Design review of the part built by this model. Coordinates are the model's own, in mm. A direction names the side the tool comes from. Give positions to 0.01 mm unless a question says otherwise; leave off trailing zeros. Loops run counter-clockwise (first coordinate to the right, second up) from the corner with the lowest first, then second, coordinate; pieces in that order, holes last. Notation, with made-up numbers: M 15,73 L 70,73 A21 ccw 70,87 Z; hole C 13.5,73.5 d11. An arc over 180 degrees is marked long. Answer as CSV lines item,"result".
```python
from build123d import *
from build123d.topology import SkipClean

# Parameters (mm, degrees)
SKETCH2_R               = 15
SKETCH2_R_2             = 11.15
BOSS_EXTRUDE1_DEPTH     = 7
SKETCH3_R               = 15
SKETCH3_R_2             = 9
BOSS_EXTRUDE2_DEPTH     = 3
BOSS_EXTRUDE3_START     = 5
SKETCH4_R               = 15
SKETCH4_R_2             = 11.15
BOSS_EXTRUDE3_DEPTH     = 5
BOSS_EXTRUDE4_DEPTH     = 8
BOSS_EXTRUDE5_START     = 20
SKETCH7_W               = 10
SKETCH7_H               = 30
BOSS_EXTRUDE5_DEPTH     = 20
BOSS_EXTRUDE6_DEPTH     = 7
SKETCH10_W              = 2
SKETCH10_H              = 90
CUT_EXTRUDE1_DEPTH      = 20
SKETCH12_R              = 2.75
CUT_EXTRUDE2_DEPTH      = 20
BOSS_EXTRUDE7_DEPTH     = 10
BOSS_EXTRUDE8_DEPTH     = 10
SKETCH15_W              = 10
SKETCH15_H              = 10
BOSS_EXTRUDE9_DEPTH     = 20
SKETCH16_W              = 10
SKETCH16_H              = 10
BOSS_EXTRUDE10_DEPTH    = 10
SKETCH17_W              = 10
SKETCH17_H              = 10
BOSS_EXTRUDE11_DEPTH    = 90
FILLET1_R               = 7.5
BOSS_EXTRUDE12_START    = 10
SKETCH18_R              = 11.15
BOSS_EXTRUDE12_DEPTH    = 10
BOSS_EXTRUDE13_START    = -3
SKETCH19_R              = 9
BOSS_EXTRUDE13_DEPTH    = 3
CUT_EXTRUDE3_DEPTH      = 88.943163464
CUT_EXTRUDE3_DEPTH_BACK = 88.943163464
SKETCH21_W              = 10
SKETCH21_H              = 10
BOSS_EXTRUDE14_DEPTH    = 20
SKETCH22_W              = 10
SKETCH22_H              = 20
BOSS_EXTRUDE15_DEPTH    = 20
FILLET2_R               = 7.5
SKETCH23_R              = 2.75
CUT_EXTRUDE4_DEPTH      = 20


with BuildPart() as part:
    # Sketch2 → Boss-Extrude1 (new body)
    with BuildSketch(Plane.XY):
        Circle(SKETCH2_R)
        Circle(SKETCH2_R_2, mode=Mode.SUBTRACT)
    extrude(amount=-BOSS_EXTRUDE1_DEPTH)

    # Sketch3 → Boss-Extrude2 (add)
    with BuildSketch(Plane(origin=(0, 0, -7), x_dir=(-1, 0, 0), z_dir=(0, 0, -1))):
        with Locations(Location((0, 0, 0), (0, 0, 180))):
            Circle(SKETCH3_R)
        Circle(SKETCH3_R_2, mode=Mode.SUBTRACT)
    extrude(amount=BOSS_EXTRUDE2_DEPTH)

    # Sketch4 → Boss-Extrude3 (add)
    with BuildSketch(Plane.XY.offset(BOSS_EXTRUDE3_START)):
        Circle(SKETCH4_R)
        Circle(SKETCH4_R_2, mode=Mode.SUBTRACT)
    extrude(amount=-BOSS_EXTRUDE3_DEPTH)

    # Sketch5 → Boss-Extrude4 (add)
    with BuildSketch(Plane.XY.offset(5)):
        with BuildLine():
            Line((0, 45), (0, 15))
            ThreePointArc((0, 15), (10.606601718, 10.606601718), (15, 0))
            ThreePointArc((15, 0), (10.606601718, -10.606601718), (0, -15))
            Line((0, -15), (0, -45))
            Line((0, -45), (17, -45))
            Line((17, -45), (17, 15))
            Line((17, 15), (17, 45))
            Line((17, 45), (0, 45))
        make_face()
    extrude(amount=-BOSS_EXTRUDE4_DEPTH)

    # Sketch7 → Boss-Extrude5 (add)
    with SkipClean():  # the faces are left unmerged after this step: merging them gives an invalid solid
        with BuildSketch(Plane.XY.offset(5).offset(BOSS_EXTRUDE5_START)):
            with Locations((12, 30)):
                Rectangle(SKETCH7_W, SKETCH7_H)
            with BuildLine():
                Line((7, -15), (17, -15))
                Line((17, -15), (17, 15))
                Line((17, 15), (7, 15))
                Line((7, 15), (7, 8.678853611))
                ThreePointArc((7, 8.678853611), (10.059137637, 4.810015592), (11.15, 0))
                ThreePointArc((11.15, 0), (10.059137637, -4.810015592), (7, -8.678853611))
                Line((7, -8.678853611), (7, -15))
            make_face()
            with Locations((12, -30)):
                Rectangle(SKETCH7_W, SKETCH7_H)
        extrude(amount=-BOSS_EXTRUDE5_DEPTH)

    # Sketch9 → Boss-Extrude6 (add)
    with SkipClean():  # the faces are left unmerged after this step: merging them gives an invalid solid
        with BuildSketch(Plane(origin=(0, 0, -3), x_dir=(-1, 0, 0), z_dir=(0, 0, -1))):
            with BuildLine():
                Line((-17, -45), (0, -45))
                Line((0, -45), (0, -15))
                ThreePointArc((0, -15), (-15, 0), (0, 15))
                Line((0, 15), (0, 45))
                Line((0, 45), (-17, 45))
                Line((-17, 45), (-17, -45))
            make_face()
        extrude(amount=BOSS_EXTRUDE6_DEPTH)

    # Sketch10 → Cut-Extrude1 (cut)
    with BuildSketch(Plane.ZY):
        with Locations((4, 0)):
            Rectangle(SKETCH10_W, SKETCH10_H)
    extrude(amount=CUT_EXTRUDE1_DEPTH, mode=Mode.SUBTRACT)

    # Sketch12 → Cut-Extrude2 (cut)
    with BuildSketch(Plane.ZY.offset(-7)):
        with Locations((15, -35.919713403)):
            Circle(SKETCH12_R)
        with Locations((15, -17.759140208)):
            Circle(SKETCH12_R)
        with Locations((15, 17.759140208)):
            Circle(SKETCH12_R)
        with BuildLine():
            ThreePointArc((17.75, 35.919713403), (16.944543648, 37.864257051), (15, 38.669713403))
            Line((15, 38.669713403), (15, 33.169713403))
            ThreePointArc((15, 33.169713403), (16.944543648, 33.975169754), (17.75, 35.919713403))
        make_face()
        with BuildLine():
            Line((15, 33.169713403), (15, 38.669713403))
            ThreePointArc((15, 38.669713403), (12.25, 35.919713403), (15, 33.169713403))
        make_face()
    extrude(amount=-CUT_EXTRUDE2_DEPTH, mode=Mode.SUBTRACT)

    # Sketch13 → Boss-Extrude7 (add)
    with BuildSketch(Plane.XZ.offset(45)):
        Polygon((7, 5), (0, 5), (0, -10), (17, -10), (17, 25), (7, 25), align=None)
    extrude(amount=BOSS_EXTRUDE7_DEPTH)

    # Sketch14 → Boss-Extrude8 (add)
    with BuildSketch(Plane(origin=(0, 45, 0), x_dir=(1, 0, 0), z_dir=(0, 1, 0))):
        Polygon((0, -5), (7, -5), (7, -25), (17, -25), (17, 10), (0, 10), align=None)
    extrude(amount=BOSS_EXTRUDE8_DEPTH)

    # Sketch15 → Boss-Extrude9 (add)
    with BuildSketch(Plane.XY.offset(25)):
        with Locations((12, 50)):
            Rectangle(SKETCH15_W, SKETCH15_H)
        with Locations((12, -50)):
            Rectangle(SKETCH15_W, SKETCH15_H)
    extrude(amount=BOSS_EXTRUDE9_DEPTH)

    # Sketch16 → Boss-Extrude10 (add)
    with BuildSketch(Plane.XY.offset(45)):
        with Locations((12, 50)):
            Rectangle(SKETCH16_W, SKETCH16_H)
        with Locations((12, -50)):
            Rectangle(SKETCH16_W, SKETCH16_H)
    extrude(amount=BOSS_EXTRUDE10_DEPTH)

    # Sketch17 → Boss-Extrude11 (add)
    with BuildSketch(Plane(origin=(0, -45, 0), x_dir=(1, 0, 0), z_dir=(0, 1, 0))):
        with Locations((12, -50)):
            Rectangle(SKETCH17_W, SKETCH17_H)
    extrude(amount=BOSS_EXTRUDE11_DEPTH)

    # Fillet1
    fillet1_edges = [part.edges().sort_by_distance(p)[0] for p in [
        (12, 45, 25),
        (12, -45, 25),
        (12, -45, 45),
        (12, 45, 45),
    ]]
    fillet(fillet1_edges, radius=FILLET1_R)

    # Sketch18 → Boss-Extrude12 (add)
    with BuildSketch(Plane.XY.offset(55).offset(BOSS_EXTRUDE12_START)):
        with BuildLine():
            ThreePointArc((0, 15), (-15, 0), (0, -15))
            Line((0, -15), (0, -55))
            Line((0, -55), (17, -55))
            Line((17, -55), (17, 55))
            Line((17, 55), (0, 55))
            Line((0, 55), (0, 15))
        make_face()
        Circle(SKETCH18_R, mode=Mode.SUBTRACT)
    extrude(amount=-BOSS_EXTRUDE12_DEPTH)

    # Sketch19 → Boss-Extrude13 (add)
    with BuildSketch(Plane(origin=(0, 0, 55), x_dir=(-1, 0, 0), z_dir=(0, 0, -1)).offset(BOSS_EXTRUDE13_START)):
        with BuildLine():
            Line((0, 15), (0, 55))
            Line((0, 55), (-17, 55))
            Line((-17, 55), (-17, -55))
            Line((-17, -55), (0, -55))
            Line((0, -55), (0, -15))
            ThreePointArc((0, -15), (15, 0), (0, 15))
        make_face()
        Circle(SKETCH19_R, mode=Mode.SUBTRACT)
    extrude(amount=BOSS_EXTRUDE13_DEPTH)

    # Sketch20 → Cut-Extrude3 (cut, two sides: drawn at the far end of the back side and taken through both)
    with BuildSketch(Plane.ZY.offset(-7).offset(-CUT_EXTRUDE3_DEPTH_BACK)):
        with BuildLine():
            ThreePointArc((51.651650429, -48.901650429), (49.954029868, -46.360981715), (46.957106781, -46.957106781))
            Line((46.957106781, -46.957106781), (50.846194078, -50.846194078))
            ThreePointArc((50.846194078, -50.846194078), (51.442319144, -49.954029868), (51.651650429, -48.901650429))
        make_face()
        with BuildLine():
            Line((50.846194078, -50.846194078), (46.957106781, -46.957106781))
            ThreePointArc((46.957106781, -46.957106781), (46.957106781, -50.846194078), (50.846194078, -50.846194078))
        make_face()
        with BuildLine():
            ThreePointArc((51.651650429, 48.901650429), (51.442319144, 49.954029868), (50.846194078, 50.846194078))
            Line((50.846194078, 50.846194078), (46.957106781, 46.957106781))
            ThreePointArc((46.957106781, 46.957106781), (49.954029868, 46.360981715), (51.651650429, 48.901650429))
        make_face()
        with BuildLine():
            Line((46.957106781, 46.957106781), (50.846194078, 50.846194078))
            ThreePointArc((50.846194078, 50.846194078), (46.957106781, 50.846194078), (46.957106781, 46.957106781))
        make_face()
    extrude(amount=CUT_EXTRUDE3_DEPTH + CUT_EXTRUDE3_DEPTH_BACK, mode=Mode.SUBTRACT)

    # Sketch21 → Boss-Extrude14 (add)
    with BuildSketch(Plane.XZ.offset(55)):
        Polygon((0, 5), (0, -10), (17, -10), (17, 5), (7, 5), align=None)
        with Locations((12, 10)):
            Rectangle(SKETCH21_W, SKETCH21_H)
    extrude(amount=BOSS_EXTRUDE14_DEPTH)

    # Sketch22 → Boss-Extrude15 (add)
    with BuildSketch(Plane.XY.offset(15)):
        with Locations((12, -65)):
            Rectangle(SKETCH22_W, SKETCH22_H)
    extrude(amount=BOSS_EXTRUDE15_DEPTH)

    # Fillet2
    fillet2_edges = [part.edges().sort_by_distance(p)[0] for p in [
        (12, -55, 35),
        (12, -75, 35),
    ]]
    fillet(fillet2_edges, radius=FILLET2_R)

    # Sketch23 → Cut-Extrude4 (cut)
    with BuildSketch(Plane.ZY.offset(-7)):
        with Locations((15, -65)):
            Circle(SKETCH23_R)
    extrude(amount=-CUT_EXTRUDE4_DEPTH, mode=Mode.SUBTRACT)


solid = part.part
```
1. We need section B-B, the plane x = -7.5. Write out the cut boundary in (y, z).
Answer block:
outline,"M -12.99,-10 L -4.97,-10 L -4.97,-7 L -8.25,-7 L -8.25,3 L -12.99,3 Z; M -12.99,55 L -4.97,55 L -4.97,58 L -8.25,58 L -8.25,65 L -12.99,65 Z; M 4.97,-10 L 12.99,-10 L 12.99,3 L 8.25,3 L 8.25,-7 L 4.97,-7 Z; M 4.97,55 L 12.99,55 L 12.99,65 L 8.25,65 L 8.25,58 L 4.97,58 Z"
2. We need section D-D, the plane x = 4. Write out the cut boundary in (y, z).
Answer block:
outline,"M -75,-10 L -8.06,-10 L -8.06,-7 L -10.41,-7 L -10.41,5 L -75,5 Z; M -55,55 L -8.06,55 L -8.06,58 L -10.41,58 L -10.41,65 L -55,65 Z; M 8.06,-10 L 55,-10 L 55,5 L 10.41,5 L 10.41,-7 L 8.06,-7 Z; M 8.06,55 L 55,55 L 55,65 L 10.41,65 L 10.41,58 L 8.06,58 Z"
3. For P1, Ø8, axis at y = 44.5, z = 59.5, coming from the -X side; P2, Ø15, axis at y = -0.5, z = 34, coming from the -X side; P3, Ø12, axis at x = -7, y = -3, coming from the +Z side; P4, Ø1.5, axis at x = 8.5, y = -1.5, coming from the +Z side, all flat-tipped, find the tip position at first contact; note any pin that passes through.
Answer block:
P1,"x = 0"
P2,"through"
P3,"z = 65"
P4,"z = 58"
4. To check wall thickness, follow L1, parallel to Z at x = 2, y = -37; L2, parallel to Z at x = 14, y = 3.5; L3, parallel to X at y = 26.5, z = 0. State the ranges of each line that lie inside material, in increasing order. Write a range as [from, to].
Answer block:
L1,"[-10, 5], [55, 65]"
L2,"[-10, 25], [45, 65]"
L3,"[0, 17]"
5. We need section A-A, the plane y = -65. Write out the cut boundary in (x, z).
Answer block:
outline,"M 0,-10 L 17,-10 L 17,12.25 L 7,12.25 L 7,5 L 0,5 Z; M 7,17.75 L 17,17.75 L 17,35 L 7,35 Z"
6. The part is to be moulded in two halves that separate along X. For faces 1 (the flat face through (8, -9, -10)), 2 (the cylindrical face through (10.635, 3.349, 61.549)), 3 (the cylindrical face through (-15, 0, 60)), say which applies: pulls with the +X half, pulls with the -X half, needs draft (parallel to the pull), parting line crosses it, or undercut.
Answer block:
face 1,"needs draft"
face 2,"undercut"
face 3,"pulls with the -X half"
7. For faces 4 (the flat face through (-0.77, 9.14, 58)), 5 (the cylindrical face through (12.07, 42.745, 42.861)), 6 (the flat face through (0.77, -9.14, -7)), 7 (the flat face through (-11, 1, 55)), list the 3-axis set-ups (+Z, -Z, +X, -X, +Y, -Y) from which the entire face can be reached by the end or side of a thin tool; tool diameter is ignored.
Answer block:
face 4,"+Z"
face 5,"+X, -X"
face 6,"none"
face 7,"-X, +Y, -Y"
8. We need section C-C, the plane z = 49.5. Write out the cut boundary in (x, y), plus the area to 3 significant figures.
Answer block:
outline,"M 7,-55 L 17,-55 L 17,-51.59 L 7,-51.59 Z; M 7,-46.22 L 17,-46.22 L 17,46.22 L 7,46.22 Z; M 7,51.59 L 17,51.59 L 17,55 L 7,55 Z"
area,"993 mm²"
